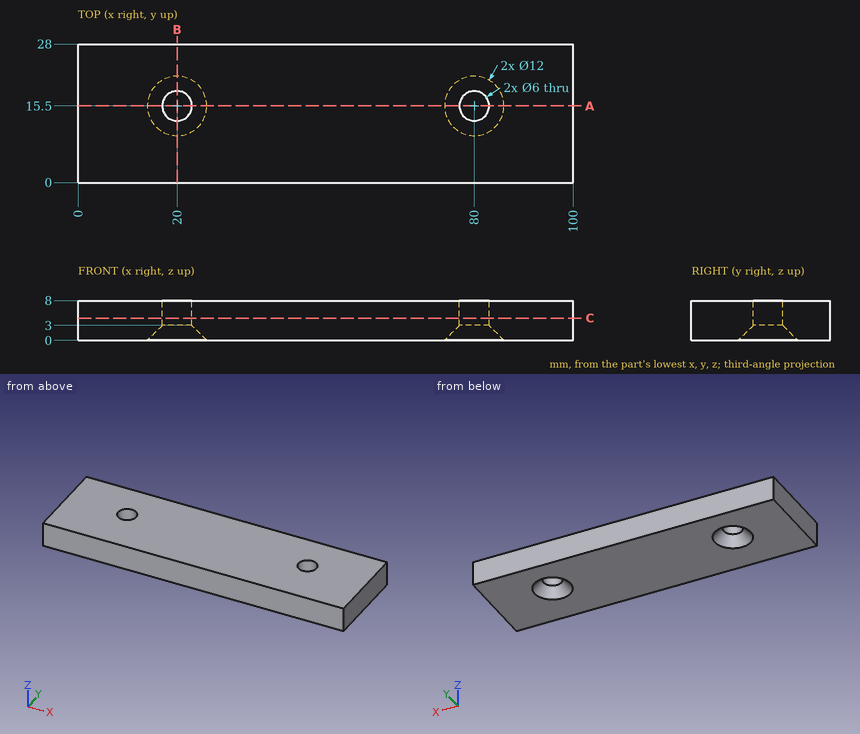
Here's the drawing with two shaded views (mm, measured from the low corner). I have some questions. Round coordinates to 2 decimals unless told otherwise and drop trailing zeros. Loops run counter-clockwise (first coordinate to the right, second up) from the corner with the lowest first, then second, coordinate; pieces in that order, holes last. Notation, with made-up numbers: (35, -21.75) - (85, -21.75) arc R8 cw to (85, -7.75) - close; hole circle Ø7 at (88.25, 86.25). An arc over 180 degrees is marked (long way). Use CSV: the item, a comma, the result in double quotes.
Item 1: If we section it at A-A on y = 15.5: List the corners of the cut face in (x, z) for me.
Here are the results:
outline,"(0, 0) - (14, 0) - (17, 3) - (17, 8) - (0, 8) - close; (23, 3) - (26, 0) - (74, 0) - (77, 3) - (77, 8) - (23, 8) - close; (83, 3) - (86, 0) - (100, 0) - (100, 8) - (83, 8) - close"
Item 2: I need wall thicknesses on L1, parallel to X at y = 15.5, z = 6.2; L2, parallel to Y at x = 20, z = 4.65; L3, parallel to X at y = 17.5, z = 4. Which ranges of each line are inside material? Lowest first, please. Write a range as [from, to].
Here are the results:
L1,"x = [0, 17], [23, 77], [83, 100]"
L2,"y = [0, 12.5], [18.5, 28]"
L3,"x = [0, 17.76], [22.24, 77.76], [82.24, 100]"
Item 3: If we section it at C-C on z = 4.5: List the corners of the cut face in (x, y) for me.
Here are the results:
outline,"(0, 0) - (100, 0) - (100, 28) - (0, 28) - close; hole circle Ø6 at (20, 15.5); hole circle Ø6 at (80, 15.5)"
Item 4: If we section it at B-B on x = 20: List the corners of the cut face in (y, z) for me.
Here are the results:
outline,"(0, 0) - (9.5, 0) - (12.5, 3) - (12.5, 8) - (0, 8) - close; (18.5, 3) - (21.5, 0) - (28, 0) - (28, 8) - (18.5, 8) - close"
